from build123d import *

# Parameters (mm, degrees)
F0_R      = 50
F1_DEPTH  = 10
F6_R      = 5
F7_DEPTH  = 7
F5_R      = 1.5
F8_DEPTH  = 17.001
F13_DEPTH = 10.001


with BuildPart() as f1:
    # F0 (on Front) → F1 (new body)
    with BuildSketch(Plane.XZ):
        Circle(F0_R)
    extrude(amount=F1_DEPTH)

    # F3 (on Right) → F4 (revolve)
    with BuildSketch(Plane.YZ):
        with BuildLine():
            Line((-10, 50), (0, 50))
            add(Edge.make_bspline(
                [(0, 50), (-2.587933, 50.855839), (-2.303226, 52.902121), (-5, 53.30912)],
                knots=[0, 0, 0, 0, 5.995855, 5.995855, 5.995855, 5.995855], degree=3))
            add(Edge.make_bspline(
                [(-10, 50), (-7.412067, 50.855839), (-7.696774, 52.902121), (-5, 53.30912)],
                knots=[0, 0, 0, 0, 5.995855, 5.995855, 5.995855, 5.995855], degree=3))
        make_face()
    revolve(axis=Axis((0, -20.942401, 0), (0, -1, 0)))

    # F6 (on face) → F7 (join)
    with BuildSketch(Plane(origin=(0, 0, 0), x_dir=(-1, 0, 0), z_dir=(0, 1, 0))):
        Circle(F6_R)
    extrude(amount=F7_DEPTH)

    # F5 (on face) → F8 (cut, through all)
    with BuildSketch(Plane.XZ.offset(10)):
        Circle(F5_R)
    extrude(amount=-F8_DEPTH, mode=Mode.SUBTRACT)

    # F9 (on Right) → F11 (revolve, cut)
    with BuildSketch(Plane.YZ):
        with BuildLine():
            Line((6, 5), (1, 5))
            ThreePointArc((1, 5), (3.5, 3.5), (6, 5))
        make_face()
    revolve(axis=Axis((0, 3.22971, 0), (0, 1, 0)), mode=Mode.SUBTRACT)

    # F12 (on face) → F13 (cut, through all)
    with BuildSketch(Plane(origin=(0, 0, 0), x_dir=(-1, 0, 0), z_dir=(0, 1, 0))):
        with BuildLine():
            Line((9.682458, 2.5), (41.925529, 2.5))
            ThreePointArc((41.925529, 2.5), (29.698485, 29.698485), (2.5, 41.925529))
            Line((2.5, 41.925529), (2.5, 9.682458))
            ThreePointArc((2.5, 9.682458), (7.071068, 7.071068), (9.682458, 2.5))
        make_face()
        with BuildLine():
            ThreePointArc((2.5, -41.925529), (29.698485, -29.698485), (41.925529, -2.5))
            Line((41.925529, -2.5), (9.682458, -2.5))
            ThreePointArc((9.682458, -2.5), (7.071068, -7.071068), (2.5, -9.682458))
            Line((2.5, -9.682458), (2.5, -41.925529))
        make_face()
        with BuildLine():
            Line((-2.5, 9.682458), (-2.5, 41.925529))
            ThreePointArc((-2.5, 41.925529), (-29.698485, 29.698485), (-41.925529, 2.5))
            Line((-41.925529, 2.5), (-9.682458, 2.5))
            ThreePointArc((-9.682458, 2.5), (-7.071068, 7.071068), (-2.5, 9.682458))
        make_face()
        with BuildLine():
            ThreePointArc((-2.5, -9.682458), (-7.071068, -7.071068), (-9.682458, -2.5))
            Line((-9.682458, -2.5), (-41.925529, -2.5))
            ThreePointArc((-41.925529, -2.5), (-29.698485, -29.698485), (-2.5, -41.925529))
            Line((-2.5, -41.925529), (-2.5, -9.682458))
        make_face()
    extrude(amount=-F13_DEPTH, mode=Mode.SUBTRACT)


solid = f1.part
Check sheet for the modelled part. Datum: model origin and axes. Units: mm. A direction names the side the tool comes from. Coordinates: 2 decimals unless noted, no trailing zeros.
Item 1: Depth check by flat-ended pin: pin 1 Ø8 at (y, z) = (-6, 18) entering from -X; pin 2 Ø3 at (x, y) = (-20.5, -4.5) entering from +Z; pin 3 Ø5 at (x, y) = (30, -4) entering from -Z. Enter the tip coordinate at first touch or a pass-through.
Numbers:
pin 1: stops at x = -51.4
pin 2: stops at z = 49.78
pin 3: stops at z = -45.55
Item 2: Cross-section at A-A on x = 19.5. Count the separate pieces of the cut face and the enclosed holes in it, then the cut area to 3 significant figures.
Numbers:
separate pieces: 3
enclosed holes: 0
area: 265 mm2
Item 3: Access from +Z, -Z, +X, -X, +Y, -Y to the whole of each face (thin tool, end or side, straight path). Record for faces 1 (the face through (26, -5, -2.5)), 2 (the face through (10, -10, 1)), 3 (the face through (-4.619, 0.493, -1.915)).
Numbers:
face 1: +Y, -Y
face 2: +Z, -Z, +X, -X, -Y
face 3: +Y
Item 4: Scan lines: probe 1 along X at (y, z) = (-1.25, 35); probe 2 along X at (y, z) = (-1.5, -35.5); probe 3 along Z at (x, y) = (-19.5, -4.5). Record each from-to range of solid material in increasing order.
Numbers:
probe 1: x = -36.58 to -23.22, -2.5 to 2.5, 23.22 to 36.58
probe 2: x = -36.37 to -22.44, -2.5 to 2.5, 22.44 to 36.37
probe 3: z = -49.5 to -37.2, -2.5 to 2.5, 37.2 to 49.5
